Check sheet for the modelled part. Datum: model origin and axes. Units: mm. Face numbers are marked on the shaded views. Give positions to 0.01 mm unless a question says otherwise; leave off trailing zeros. Order: outer loops, then holes, each group sorted by start corner. A loop starts at its lowest first (then second) coordinate and runs counter-clockwise, first axis right, second up. Notation, with made-up numbers: (65.5, 24) -> (79.5, 24) arc R21 ccw to (79.5, 52) -> close; hole circle Ø5 at (61, 33). An arc over 180 degrees is marked (long way). One line per question, with ' | ' between items.
```python
from build123d import *

# Parameters (mm, degrees)
F0_R     = 2
F0_R_2   = 1.5
F1_DEPTH = 5


with BuildPart() as f1:
    # F0 (on Front) → F1 (new body)
    with BuildSketch(Plane.XZ):
        with BuildLine():
            ThreePointArc((20, -11.5), (20.732233, -13.267767), (22.5, -14))
            Line((22.5, -14), (24.166667, -14))
            ThreePointArc((24.166667, -14), (25.701518, -13.473381), (26.589744, -12.115385))
            Line((26.589744, -12.115385), (26.780755, -11.363276))
            ThreePointArc((26.780755, -11.363276), (27.747195, -9.946861), (29.398892, -9.486282))
            ThreePointArc((29.398892, -9.486282), (34.111538, -6.107692), (31.582114, -0.889847))
            ThreePointArc((31.582114, -0.889847), (30.350345, 0.303041), (30.176878, 2.008956))
            Line((30.176878, 2.008956), (37.830769, 32.146154))
            ThreePointArc((37.830769, 32.146154), (36.025514, 37.721463), (30.21772, 38.504118))
            Line((30.21772, 38.504118), (22.403935, 34.940405))
            ThreePointArc((22.403935, 34.940405), (21.76066, 34.516571), (21.276965, 33.917007))
            Line((21.276965, 33.917007), (11.08563, 16.287694))
            ThreePointArc((11.08563, 16.287694), (10.835365, 15.684211), (10.75, 15.036493))
            Line((10.75, 15.036493), (10.75, 11.5))
            ThreePointArc((10.75, 11.5), (10.017767, 9.732233), (8.25, 9))
            Line((8.25, 9), (0, 9))
            Line((0, 9), (0, 0))
            Line((0, 0), (17.5, 0))
            ThreePointArc((17.5, 0), (19.267767, -0.732233), (20, -2.5))
            Line((20, -2.5), (20, -11.5))
        make_face()
        with Locations((15.25, 5)):
            Circle(F0_R, mode=Mode.SUBTRACT)
        with Locations((23, -10)):
            Circle(F0_R_2, mode=Mode.SUBTRACT)
        with Locations((29.75, -5)):
            Circle(F0_R, mode=Mode.SUBTRACT)
        with Locations((26, 6.5)):
            Circle(F0_R_2, mode=Mode.SUBTRACT)
        with Locations((15.25, 14.5)):
            Circle(F0_R, mode=Mode.SUBTRACT)
        with Locations((24.5, 31.5)):
            Circle(F0_R_2, mode=Mode.SUBTRACT)
        with Locations((32.5, 33.5)):
            Circle(F0_R_2, mode=Mode.SUBTRACT)
    extrude(amount=F1_DEPTH)

    # F2: F1 across plane


with BuildPart() as f1_1:
    add(f1.part)
    add(f1.part.mirror(Plane.YZ))


solid = f1_1.part
```
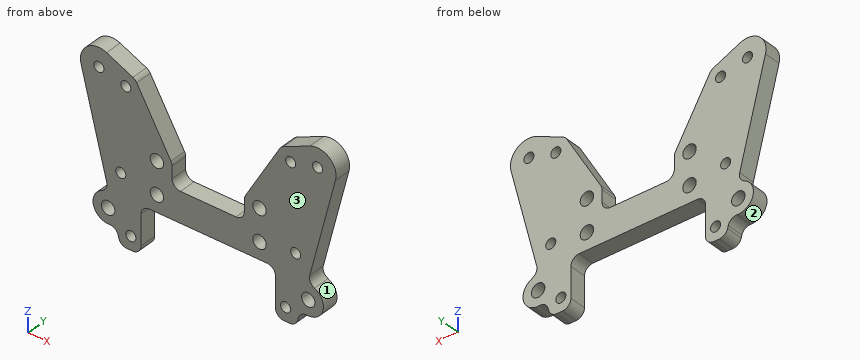
Q1. Depth check by flat-ended pin: pin 1 Ø3.5 at (x, z) = (29.75, -5) entering from -Y; pin 2 Ø1.1 at (y, z) = (-2, 13.5) entering from -X; pin 3 Ø1 at (x, y) = (25.5, -3) entering from +Z; pin 4 Ø3 at (y, z) = (-3.5, 14) entering from +X. Enter the tip coordinate at first touch or a pass-through.
Result sheet:
pin 1: passes through | pin 2: stops at x = -33.23 | pin 3: stops at z = 36.58 | pin 4: stops at x = 33.6
Q2. Section check A-A (z = 18). Enter the section's corners in (x, y), and give its area (3 significant figures).
Result sheet:
outline: (-34.24, -5) -> (-12.08, -5) -> (-12.08, 0) -> (-34.24, 0) -> close; (12.08, -5) -> (34.24, -5) -> (34.24, 0) -> (12.08, 0) -> close | area: 222 mm2
Q3. Section check D-D (x = -32.5). Enter the section's corners in (y, z).
Result sheet:
outline: (-5, -8.56) -> (0, -8.56) -> (0, -1.44) -> (-5, -1.44) -> close; (-5, 11.16) -> (0, 11.16) -> (0, 32) -> (-5, 32) -> close; (-5, 35) -> (0, 35) -> (0, 39) -> (-5, 39) -> close
Q4. Section check B-B (x = -15.25). Enter the section's corners in (y, z).
Result sheet:
outline: (-5, 0) -> (0, 0) -> (0, 3) -> (-5, 3) -> close; (-5, 7) -> (0, 7) -> (0, 12.5) -> (-5, 12.5) -> close; (-5, 16.5) -> (0, 16.5) -> (0, 23.49) -> (-5, 23.49) -> close
Q5. Mould release check, pull along Z, two halves, no side actions. Record for the marked faces 1, 2 and 3: pulls with the +Z half, pulls with the -Z half, needs draft (parallel to the pull), parting line crosses it, or undercut.
Result sheet:
face 1: undercut | face 2: undercut | face 3: needs draft
Q6. Section check C-C (z = -6). Enter the section's corners in (x, y), and give its area (3 significant figures).
Result sheet:
outline: (-34.14, -5) -> (-31.48, -5) -> (-31.48, 0) -> (-34.14, 0) -> close; (-28.02, -5) -> (-20, -5) -> (-20, 0) -> (-28.02, 0) -> close; (20, -5) -> (28.02, -5) -> (28.02, 0) -> (20, 0) -> close; (31.48, -5) -> (34.14, -5) -> (34.14, 0) -> (31.48, 0) -> close | area: 107 mm2
Q7. Thickness scan on line 1 (X direction, y = -3.2, z = 7.5); line 2 (Z direction, x = -17, y = -1.5); line 3 (Z direction, x = 16, y = -4.7). Record the ranges inside material, lowest first.
Result sheet:
line 1: x = -31.57 to -27.12, -24.88 to 24.88, 27.12 to 31.57 | line 2: z = 0 to 4.03, 5.97 to 13.53, 15.47 to 26.52 | line 3: z = 0 to 3.15, 6.85 to 12.65, 16.35 to 24.79
